Can you work these out from the model? Positions are in its coordinate system, mm. Coordinates: 2 decimals unless noted, no trailing zeros. Order: outer loops, then holes, each group sorted by start corner. A loop starts at its lowest first (then second) coordinate and runs counter-clockwise, first axis right, second up. Notation, with made-up numbers: (-30, -24.5) -> (22, -24.5) arc R16 cw to (22, -19.5) -> close; hole circle Ø5 at (5.25, 73.25). An arc over 180 degrees is marked (long way). Answer as CSV lines item,"result".
from build123d import *

# Parameters (mm, degrees)
SKETCH1_R              = 2
BOSS_EXTRUDE1_DEPTH    = 4
BOSS_EXTRUDE1_2_DEPTH  = 4
BOSS_EXTRUDE1_3_DEPTH  = 4
BOSS_EXTRUDE1_4_DEPTH  = 4
SKETCH2_W              = 50
SKETCH2_H              = 30
BOSS_EXTRUDE2_DEPTH    = 2
F_00_CLEARANCE_HOLE2_D = 1.397
SKETCH9_R              = 2.5
BOSS_EXTRUDE3_DEPTH    = 3
F_4_CLEARANCE_HOLE1_D  = 3.2639


with BuildPart() as part:
    # Sketch1 → Boss-Extrude1 (new body)
    with BuildSketch(Plane(origin=(0, 0, 0), x_dir=(1, 0, 0), z_dir=(0, 1, 0))):
        with Locations(Location((3.75, 26.25, 0), (0, 0, 270))):
            Circle(SKETCH1_R)
    extrude(amount=BOSS_EXTRUDE1_DEPTH)



with BuildPart() as body_2:
    # Sketch1 → Boss-Extrude1 2 (new body)
    with BuildSketch(Plane(origin=(0, 0, 0), x_dir=(1, 0, 0), z_dir=(0, 1, 0))):
        with Locations(Location((46.25, 26.25, 0), (0, 0, 270))):
            Circle(SKETCH1_R)
    extrude(amount=BOSS_EXTRUDE1_2_DEPTH)


with BuildPart() as body_3:
    # Sketch1 → Boss-Extrude1 3 (new body)
    with BuildSketch(Plane(origin=(0, 0, 0), x_dir=(1, 0, 0), z_dir=(0, 1, 0))):
        with Locations(Location((46.25, 8.75, 0), (0, 0, 270))):
            Circle(SKETCH1_R)
    extrude(amount=BOSS_EXTRUDE1_3_DEPTH)


with BuildPart() as body_4:
    # Sketch1 → Boss-Extrude1 4 (new body)
    with BuildSketch(Plane(origin=(0, 0, 0), x_dir=(1, 0, 0), z_dir=(0, 1, 0))):
        with Locations(Location((3.75, 8.75, 0), (0, 0, 270))):
            Circle(SKETCH1_R)
    extrude(amount=BOSS_EXTRUDE1_4_DEPTH)


with BuildPart() as part_1:
    add(part.part)

    add(body_2.part)  # Boss-Extrude2 merges body 2

    add(body_3.part)  # Boss-Extrude2 merges body 3

    add(body_4.part)  # Boss-Extrude2 merges body 4
    # Sketch2 → Boss-Extrude2 (add)
    with BuildSketch(Plane(origin=(0, 0, 0), x_dir=(1, 0, 0), z_dir=(0, 1, 0))):
        with Locations((25, 15)):
            Rectangle(SKETCH2_W, SKETCH2_H)
    extrude(amount=-BOSS_EXTRUDE2_DEPTH)

    # #00 Clearance Hole2 (through all)
    with Locations(Plane(origin=(0, 4, 0), x_dir=(1, 0, 0), z_dir=(0, 1, 0))):
        with Locations((3.75, 26.25), (46.25, 26.25), (46.25, 8.75), (3.75, 8.75)):
            Hole(F_00_CLEARANCE_HOLE2_D / 2)

    # Sketch9 → Boss-Extrude3 (add)
    with BuildSketch(Plane.XZ.offset(2)):
        with Locations(Location((3.905878753, -3.75, 0), (0, 0, 90))):
            Circle(SKETCH9_R)
        with Locations(Location((43.905878753, -3.75, 0), (0, 0, 90))):
            Circle(SKETCH9_R)
    extrude(amount=BOSS_EXTRUDE3_DEPTH)

    # #4 Clearance Hole1 (through all)
    with Locations(Plane(origin=(0, -5, 0), x_dir=(-1, 0, 0), z_dir=(0, -1, 0))):
        with Locations((-3.905878753, 3.75), (-43.905878753, 3.75)):
            Hole(F_4_CLEARANCE_HOLE1_D / 2)


solid = part_1.part
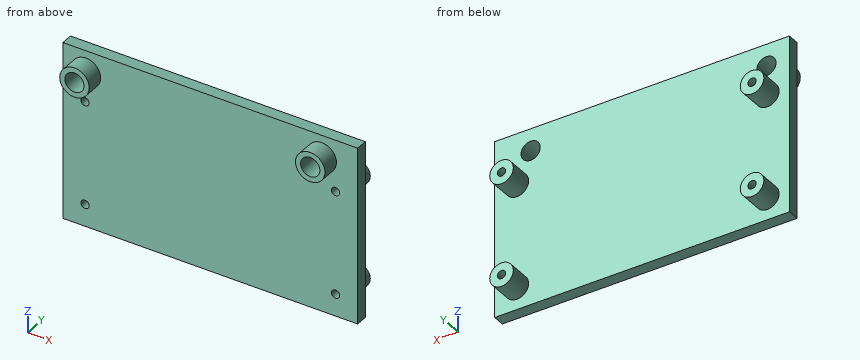
Q1. Imagine slicing it at B-B (y = 2). List the corners of the cut face in (x, z) for me, and give its area (3 significant figures).
Solution:
outline,"circle Ø4 at (3.75, -26.25); circle Ø4 at (3.75, -8.75); circle Ø4 at (46.25, -26.25); circle Ø4 at (46.25, -8.75); hole circle Ø1.4 at (3.75, -26.25); hole circle Ø1.4 at (3.75, -8.75); hole circle Ø1.4 at (46.25, -26.25); hole circle Ø1.4 at (46.25, -8.75)"
area,"44.1 mm2"
Q2. For P1, Ø2, axis at x = 34.5, z = -3.5, coming from the -Y side; P2, Ø5, axis at x = 17, y = -4, coming from the +Z side; P3, Ø9, axis at x = 20.5, z = -9, coming from the +Y side; P4, Ø1.3, axis at x = 46.25, z = -8.75, coming from the -Y side, each with a flat end and sliding along its axis, tell me the tip position at first contact or that it passes through.
Solution:
P1,"y = -2"
P2,"z = 0"
P3,"y = 0"
P4,"through"
Q3. If I drill on line 1 (Z direction, x = 3.75, y = -0.15); line 2 (X direction, y = 1.4, z = -26.25); line 3 (Z direction, x = 46, y = 1.75), over which ranges is the centre line in solid material (lowest first)?
Solution:
line 1,"-30 to -26.95, -25.55 to -9.45, -8.05 to -5.37, -2.13 to 0"
line 2,"1.75 to 3.05, 4.45 to 5.75, 44.25 to 45.55, 46.95 to 48.25"
line 3,"-28.23 to -26.9, -25.6 to -24.27, -10.73 to -9.4, -8.1 to -6.77"
Q4. Imagine slicing it at D-D (z = -3.75). List the corners of the cut face in (x, y) for me, and give its area (3 significant figures).
Solution:
outline,"(0, -2) -> (1.41, -2) -> (1.41, -5) -> (2.27, -5) -> (2.27, 0) -> (0, 0) -> close; (5.54, -5) -> (6.41, -5) -> (6.41, -2) -> (41.41, -2) -> (41.41, -5) -> (42.27, -5) -> (42.27, 0) -> (5.54, 0) -> close; (45.54, -5) -> (46.41, -5) -> (46.41, -2) -> (50, -2) -> (50, 0) -> (45.54, 0) -> close"
area,"97.4 mm2"
Q5. Imagine slicing it at A-A (z = -26.25). List the corners of the cut face in (x, y) for me, and give its area (3 significant figures).
Solution:
outline,"(0, -2) -> (3.05, -2) -> (3.05, 4) -> (1.75, 4) -> (1.75, 0) -> (0, 0) -> close; (4.45, -2) -> (45.55, -2) -> (45.55, 4) -> (44.25, 4) -> (44.25, 0) -> (5.75, 0) -> (5.75, 4) -> (4.45, 4) -> close; (46.95, -2) -> (50, -2) -> (50, 0) -> (48.25, 0) -> (48.25, 4) -> (46.95, 4) -> close"
area,"115 mm2"
Q6. Imagine slicing it at C-C (y = -1.5). List the corners of the cut face in (x, z) for me, and give its area (3 significant figures).
Solution:
outline,"(0, -30) -> (50, -30) -> (50, 0) -> (0, 0) -> close; hole circle Ø3.26 at (3.91, -3.75); hole circle Ø1.4 at (3.75, -26.25); hole circle Ø1.4 at (3.75, -8.75); hole circle Ø3.26 at (43.91, -3.75); hole circle Ø1.4 at (46.25, -26.25); hole circle Ø1.4 at (46.25, -8.75)"
area,"1,480 mm2"
